Can you work these out from the drawing? Everything is in mm from the part's minimum corner. Coordinates: 2 decimals unless noted, no trailing zeros. Loops run counter-clockwise (first coordinate to the right, second up) from the corner with the lowest first, then second, coordinate; pieces in that order, holes last. Notation, with made-up numbers: (-26.75, 58) - (-19.75, 58) arc R18 cw to (-19.75, 92) - close; hole circle Ø6 at (-27, 28). An arc over 180 degrees is marked (long way). Put each result on its own line as item: value. Start each with the question number.
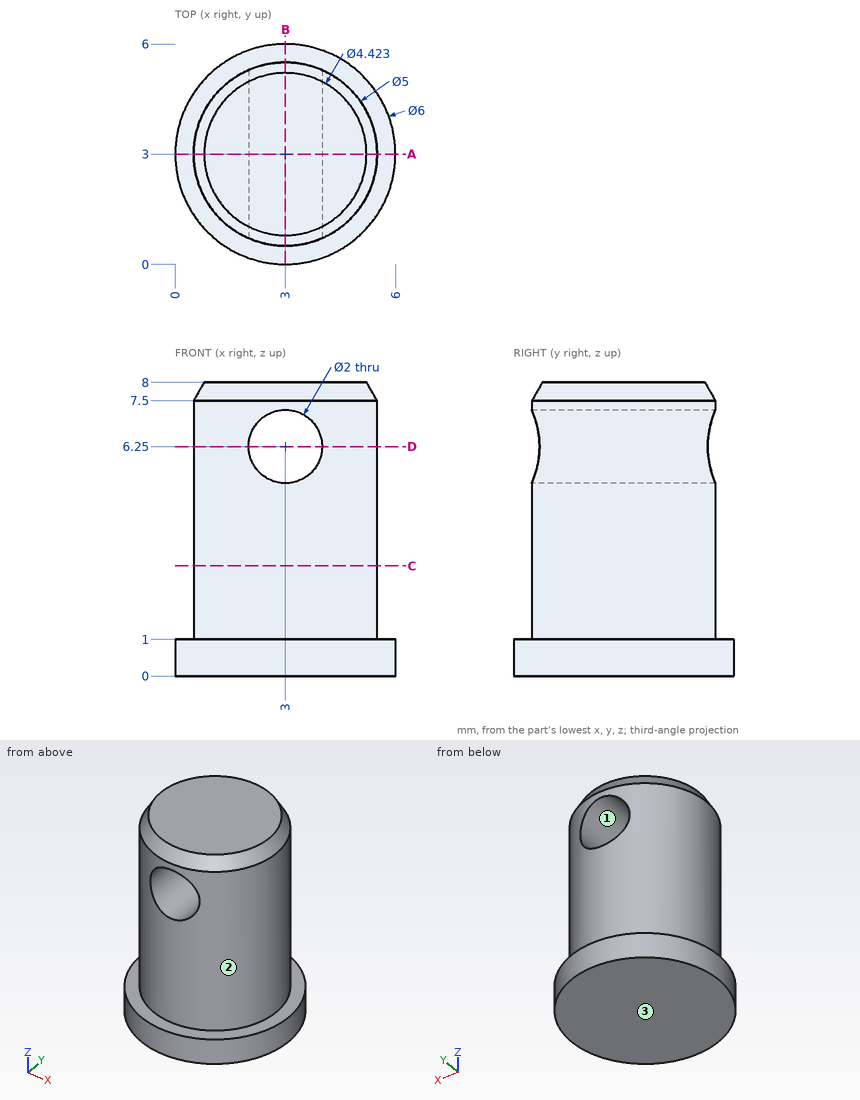
Q1. I want a section at B-B on x = 3. List the corners of the cut face in (y, z) for me.
Q2. Please list where these lines run through material, in increasing order: line 1 along Z through (x, y) = (3, 1.95); line 2 along Y through (x, z) = (2.9, 0.75); line 3 along X through (y, z) = (3.85, 6.25). Write a range as [from, to].
Q3. Will these pins go through, and if not, where does the flat tip stop? pin 1 (2.5 mm diameter, centred on x = 3, z = 6.25, fed in from +Y); pin 2 (3 mm diameter, centred on y = 5, z = 4.5, fed in from -X); pin 3 (1.5 mm diameter, centred on x = 2.5, z = 7, fed in from -Y).
Q4. I want a section at D-D on z = 6.25. List the corners of the cut face in (x, y) for me.
Q5. I want a section at C-C on z = 3. List the corners of the cut face in (x, y) for me, and give its area (3 significant figures).
Q6. We'd pull the mould along X, two halves only. Please class the marked faces 1, 2 and 3: released by +X, released by -X, zero draft, split by the parting line, or undercut.
Q7. I want a section at A-A on y = 3. List the corners of the cut face in (x, z) for me, and give its area (3 significant figures).
Calculated:
1. outline: (0, 0) - (6, 0) - (6, 1) - (5.5, 1) - (5.5, 5.25) - (0.5, 5.25) - (0.5, 1) - (0, 1) - close; (0.5, 7.25) - (5.5, 7.25) - (5.5, 7.5) - (5.21, 8) - (0.79, 8) - (0.5, 7.5) - close
2. line 1: [0, 5.25], [7.25, 8]
2. line 2: [0, 6]
2. line 3: [0.65, 2], [4, 5.35]
3. pin 1: y = 5.5
3. pin 2: x = 0.55
3. pin 3: y = 0.5
4. outline: (2, 0.71) - (2, 5.29) arc R2.5 ccw to start; (4, 0.71) arc R2.5 ccw to (4, 5.29) - close
5. outline: circle Ø5 at (3, 3)
5. area: 19.6 mm2
6. face 1: undercut
6. face 2: split by the parting line
6. face 3: zero draft
7. outline: (0, 0) - (6, 0) - (6, 1) - (5.5, 1) - (5.5, 7.5) - (5.21, 8) - (0.79, 8) - (0.5, 7.5) - (0.5, 1) - (0, 1) - close; hole circle Ø2 at (3, 6.25)
7. area: 37.7 mm2
